Autodesk Inventor part; units mm, degrees
ref_plane "YZ Plane" through (0, 0, 0) normal (1, 0, 0) x (0, 1, 0)
ref_plane "XZ Plane" through (0, 0, 0) normal (0, 1, 0) x (-1, 0, 0)
ref_plane "XY Plane" through (0, 0, 0) normal (0, 0, 1) x (1, 0, 0)
sketch "Sketch1" plane through (0, 0, 0) normal (0, 0, 1) x (1, 0, 0)
  line L0 (0, 0) -> (45, 0)
  line L1 (0, 0) -> (0, 65)
  line L2 (0, 65) -> (10, 65)
  line L3 (10, 65) -> (10, 16)
  line L4 (10, 16) -> (22.5, 16)
  line L5 (22.5, 71) -> (22.5, -20)
  line L6 (45, 0) -> (45, 65)
  line L7 (45, 65) -> (35, 65)
  line L8 (35, 65) -> (35, 16)
  line L9 (35, 16) -> (22.5, 16)
  dimension "d1" = 45
  dimension "d2" = 65
  dimension "d3" = 10
  dimension "d4" = 16
  dimension "d5" = 22.5
extrude "Extrusion1" add sketch "Sketch1" along normal mid plane 40
sketch "Sketch2" plane through (0, 0, 20) normal (0, -1, 0) x (1, 0, 0)
  circle A0 centre (22.5, -20) radius 16
  line L0 (0, 0) -> (45, 0)
  line L1 (0, -40) -> (0, 0)
  point P0 (0, -20)
  dimension "d8" = 32
  dimension "d9" = 20
  dimension "d10" = 22.5
extrude "Extrusion2" add sketch "Sketch2" along normal blind 4
fillet "Fillet1" radius 20 4 edges at (5, 65, -20) (5, 65, 20) (40, 65, 20) (40, 65, -20)
sketch "Sketch3" plane through (22.5, -4, 0) normal (0, -1, 0) x (1, 0, 0)
  circle A0 centre (0, 0) radius 16
  circle A1 centre (0, 0) radius 8
  point P0 (-22.5, 0)
  dimension "d14" = 16
extrude "Extrusion3" cut sketch "Sketch3" against normal through all contours A1
sketch "Sketch4" plane through (0, 0, -20) normal (-1, 0, 0) x (0, 0, 1)
  circle A0 centre (20, 45) radius 16
  line L0 (4, -4) -> (36, -4)
  line L1 (40, 45) -> (40, 0)
  point P0 (20, 0)
  dimension "d17" = 32
  dimension "d18" = 49
  dimension "d19" = 20
extrude "Extrusion4" add sketch "Sketch4" along normal blind 4
sketch "Sketch5" plane through (45, 0, 20) normal (1, 0, 0) x (0, 0, -1)
  circle A0 centre (20, 45) radius 16
  line L0 (4, -4) -> (36, -4)
  line L1 (0, 0) -> (0, 45)
  point P0 (20, 0)
  dimension "d22" = 32
  dimension "d23" = 49
  dimension "d24" = 20
extrude "Extrusion5" add sketch "Sketch5" along normal blind 4
sketch "Sketch6" plane through (-4, 45, 0) normal (-1, 0, 0) x (0, 0, 1)
  circle A0 centre (0, 0) radius 16
  circle A1 centre (0, 0) radius 10
  circle A2 centre (0, -35) radius 2.5
  line L0 (-20, -45) -> (20, -45)
  line L1 (-20, -45) -> (-20, 0)
  point P0 (0, -45)
  dimension "d27" = 20
  dimension "d28" = 5
  dimension "d29" = 10
  dimension "d30" = 20
extrude "Extrusion6" cut sketch "Sketch6" against normal through all contours A1 | A2
equation "\"d5\" = 0.5 * d1"
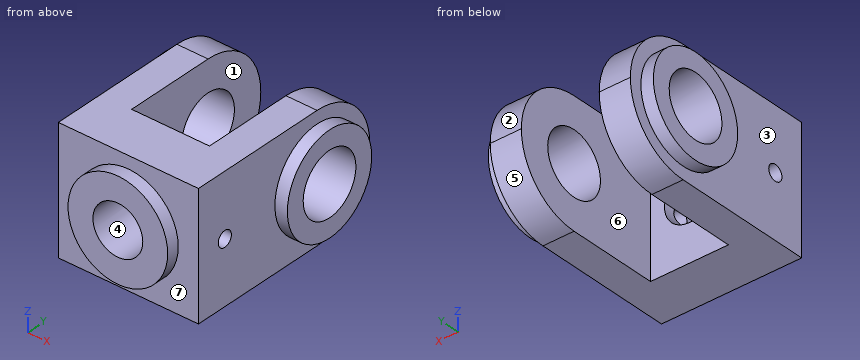
Can you work these out from the model? Positions are in its coordinate system, mm. Face numbers are marked on the shaded views. A direction names the side the tool comes from. Give positions to 0.01 mm unless a question says otherwise; leave off trailing zeros. Loops run counter-clockwise (first coordinate to the right, second up) from the corner with the lowest first, then second, coordinate; pieces in that order, holes last. Notation, with made-up numbers: (79, 9) - (114, 9) arc R15 ccw to (114, 16) - close; hole circle Ø7 at (59.5, 52.25). An arc over 180 degrees is marked (long way). Return JSON: item names as keys, results as strings.
1. I want a section at C-C on y = 44. Please give me the cut outline in (x, z), and give its area (3 significant figures).
Output values:
{"outline": "(-4, -15.97) - (0, -15.97) - (0, -20) - (10, -20) - (10, -9.95) - (-4, -9.95) - close; (-4, 9.95) - (10, 9.95) - (10, 20) - (0, 20) - (0, 15.97) - (-4, 15.97) - close; (35, -20) - (45, -20) - (45, -15.97) - (49, -15.97) - (49, -9.95) - (35, -9.95) - close; (35, 9.95) - (49, 9.95) - (49, 15.97) - (45, 15.97) - (45, 20) - (35, 20) - close", "area": "498 mm²"}
2. I'm going to push flat-ended pins straight in: pin 1 Ø8 at (y, z) = (10, 0) entering from +X; pin 2 Ø12 at (x, y) = (6.5, 52) entering from -Z (3 decimals); pin 3 Ø1.5 at (x, z) = (15, 15.5) entering from -Y. Where does each tip first touch, or does it pass through?
Output values:
{"pin 1": "stops at x = 45", "pin 2": "stops at z = -19.975", "pin 3": "stops at y = 0"}
3. I want a section at B-B on x = 22.5. Please give me the cut outline in (y, z).
Output values:
{"outline": "(-4, -16) - (0, -16) - (0, -20) - (16, -20) - (16, -8) - (-4, -8) - close; (-4, 8) - (16, 8) - (16, 20) - (0, 20) - (0, 16) - (-4, 16) - close"}
4. If I drill on line 1 (Z direction, x = 38.5, y = 10); line 2 (Y direction, x = 37, z = 0); line 3 (Y direction, x = 40, z = 0), over which ranges is the centre line in solid material (lowest first)?
Output values:
{"line 1": "z = -20 to -2.5, 2.5 to 20", "line 2": "y = -4 to 7.5, 12.5 to 35, 55 to 65", "line 3": "y = 0 to 7.5, 12.5 to 35, 55 to 65"}
5. We'd pull the mould along X, two halves only. Please class the marked faces 1, 2, 3 and 4: +X half, -X half, draft (parallel to the pull), parting line (faces both ways), or undercut.
Output values:
{"face 1": "undercut", "face 2": "draft", "face 3": "-X half", "face 4": "undercut"}
6. I want a section at A-A on y = 10. Please give me the cut outline in (x, z), and give its area (3 significant figures).
Output values:
{"outline": "(0, -20) - (45, -20) - (45, -2.5) - (30.1, -2.5) arc R8 cw to (14.9, -2.5) - (0, -2.5) - close; (0, 2.5) - (14.9, 2.5) arc R8 cw to (30.1, 2.5) - (45, 2.5) - (45, 20) - (0, 20) - close", "area": "1,450 mm²"}
7. I want a section at D-D on x = 37.5. Give the number of separate pieces and of enclosed holes in the cut face, and give its area (3 significant figures).
Output values:
{"separate pieces": "1", "enclosed holes": "2", "area": "2,140 mm²"}
8. For the marked faces 5, 6 and 7, which set-ups out of +Z, -Z, +X, -X, +Y, -Y let a thin tool reach every point of the face, with its end or its side?
Output values:
{"face 5": "-Z, +X, -X, +Y", "face 6": "+Z, -Z, +Y", "face 7": "-Y"}
